from build123d import *

# Parameters (mm, degrees)
CUT_EXTRUDE_1_DEPTH = 1
CHAMFER_2_SIZE      = 0.3


with BuildPart() as part:
    # 草图1 → 旋转1 (revolve)
    with BuildSketch(Plane(origin=(0, 0, 0), x_dir=(0, 0, -1), z_dir=(1, 0, 0)), mode=Mode.PRIVATE) as revolve_1_sk:
        with BuildLine():
            Line((0, 1.5), (0, 2.85))
            Line((0, 2.85), (-0.35, 2.85))
            ThreePointArc((-0.35, 2.85), (-1.098097646, 2.229807704), (-1.65, 1.43))
            Line((-1.65, 1.43), (-1.65, 0))
            Line((-1.65, 0), (0, 0))
            Line((0, 0), (37.3, 0))
            Line((37.3, 0), (37.3, 1.5))
            Line((37.3, 1.5), (0, 1.5))
        make_face()
    revolve(revolve_1_sk.sketch.rotate(Axis((0, 0, 0), (0, 0, -1)), 90), axis=Axis((0, 0, 0), (0, 0, -1)))

    # 草图2 → 切除-拉伸1 (cut)
    with BuildSketch(Plane.XY.offset(1.65)):
        Polygon((-0.577350269, 1), (-1.154700538, 0), (-0.577350269, -1), (0.577350269, -1), (1.154700538, 0), (0.577350269, 1), align=None)
    extrude(amount=-CUT_EXTRUDE_1_DEPTH, mode=Mode.SUBTRACT)

    # 倒角2
    chamfer_2_edges = [part.edges().sort_by_distance(p)[0] for p in [
        (-1.5, 0, -37.3),
    ]]
    chamfer(chamfer_2_edges, length=CHAMFER_2_SIZE)


solid = part.part
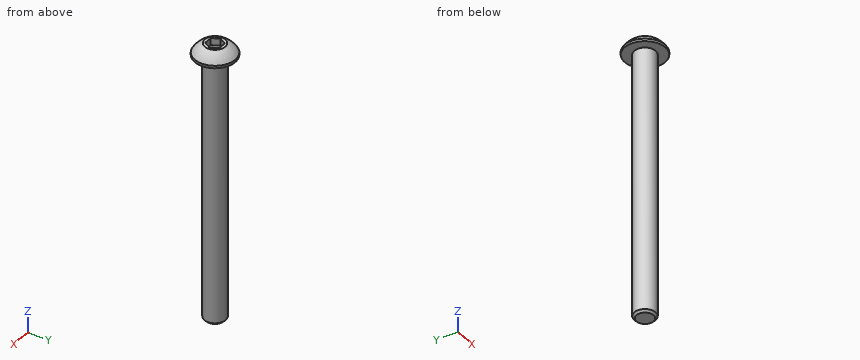
Model file for the job. Use its own axes, mm. Coordinates: 2 decimals unless noted, no trailing zeros. Loops run counter-clockwise (first coordinate to the right, second up) from the corner with the lowest first, then second, coordinate; pieces in that order, holes last. Notation, with made-up numbers: (55.25, 24.25) -> (95.25, 24.25) arc R11 ccw to (95.25, 31.25) -> close; hole circle Ø10 at (19, 56). An arc over 180 degrees is marked (long way). Use one line per item in the form item = value. Start each with the question number.
(1) Cut at A-A on z = -4.5. Give the cut face in (x, y), and give its area (3 significant figures).
(2) Flat gauge pins, fed straight in: pin 1 (1.5 mm diameter, centred on x = 1, z = -4, fed in from +Y); pin 2 (0.5 mm diameter, centred on x = 0, z = 1, fed in from -Y); pin 3 (1.5 mm diameter, centred on y = -0.5, z = -17, fed in from -X). Where does each tip first touch, or does it go through?
(3) Probe probe 1 along Y at (x, z) = (-0.95, -19); probe 2 along Z at (x, y) = (-0.2, -0.6); probe 3 along Y at (x, z) = (0.1, -5). List the from-to ranges inside material, lowest first. Write a range as from..to.
Values:
q1.outline = circle Ø3 at (0, 0)
q1.area = 7.07 mm2
q2.pin_1 = 1.48
q2.pin_2 = -2.56
q2.pin_3 = -1.5
q3.probe_1 = -1.16..1.16
q3.probe_2 = -37.3..0.65
q3.probe_3 = -1.5..1.5
